from build123d import *

# Parameters (mm, degrees)
F0_W      = 30.48
F0_H      = 15.24
F2_DEPTH  = 3.175
F1_R      = 2.413
F3_DEPTH  = 1.905
F5_R      = 1.27
F6_DEPTH  = 4.699
F4_W      = 27.94
F4_H      = 12.7
F4_R      = 3.175
F7_DEPTH  = 2.159
F8_DEPTH  = 4.699
F9_DEPTH  = 4.699
F4_R_2    = 2.54
F10_DEPTH = 2.159
F11_DEPTH = 2.159
F12_DEPTH = 2.159


with BuildPart() as f2:
    # F0 (on Top) → F2 (new body)
    with BuildSketch(Plane.XY):
        with Locations((-38.230583, 21.220251)):
            Rectangle(F0_W, F0_H)
    extrude(amount=-F2_DEPTH)

    # F1 (on face) → F3 (join)
    with BuildSketch(Plane.XY):
        with Locations((-26.800583, 25.030251)):
            Circle(F1_R)
        with Locations((-26.800583, 17.410251)):
            Circle(F1_R)
        with Locations((-34.420583, 25.030251)):
            Circle(F1_R)
        with Locations((-34.420583, 17.410251)):
            Circle(F1_R)
        with Locations((-42.040583, 25.030251)):
            Circle(F1_R)
        with Locations((-42.040583, 17.410251)):
            Circle(F1_R)
        with Locations((-49.660583, 25.030251)):
            Circle(F1_R)
        with Locations((-49.660583, 17.410251)):
            Circle(F1_R)
    extrude(amount=F3_DEPTH)

    # F5 (on face) → F6 (cut)
    with BuildSketch(Plane(origin=(0, 0, -3.175), x_dir=(1, 0, 0), z_dir=(0, 0, -1))):
        with Locations((-26.800583, -25.030251)):
            Circle(F5_R)
        with Locations((-34.420583, -25.030251)):
            Circle(F5_R)
        with Locations((-42.040583, -25.030251)):
            Circle(F5_R)
        with Locations((-49.660583, -25.030251)):
            Circle(F5_R)
        with Locations((-26.800583, -17.410251)):
            Circle(F5_R)
        with Locations((-34.420583, -17.410251)):
            Circle(F5_R)
        with Locations((-42.040583, -17.410251)):
            Circle(F5_R)
        with Locations((-49.660583, -17.410251)):
            Circle(F5_R)
    extrude(amount=-F6_DEPTH, mode=Mode.SUBTRACT)

    # F4 (on face) → F7 (cut)
    with BuildSketch(Plane(origin=(0, 0, -3.175), x_dir=(1, 0, 0), z_dir=(0, 0, -1))):
        with Locations((-38.230583, -21.220251)):
            Rectangle(F4_W, F4_H)
        with Locations((-45.850583, -21.220251)):
            Circle(F4_R, mode=Mode.SUBTRACT)
        with Locations((-38.230583, -21.220251)):
            Circle(F4_R, mode=Mode.SUBTRACT)
        with Locations((-30.610583, -21.220251)):
            Circle(F4_R, mode=Mode.SUBTRACT)
    extrude(amount=-F7_DEPTH, mode=Mode.SUBTRACT)

    # F5 (on face) → F8 (join)
    with BuildSketch(Plane(origin=(0, 0, -3.175), x_dir=(1, 0, 0), z_dir=(0, 0, -1))):
        with Locations((-49.660583, -25.030251)):
            Circle(F5_R)
    extrude(amount=-F8_DEPTH)

    # F5 (on face) → F9 (cut)
    with BuildSketch(Plane(origin=(0, 0, -3.175), x_dir=(1, 0, 0), z_dir=(0, 0, -1))):
        with Locations((-49.660583, -25.030251)):
            Circle(F5_R)
    extrude(amount=-F9_DEPTH, mode=Mode.SUBTRACT)

    # F4 (on face) → F10 (cut)
    with BuildSketch(Plane(origin=(0, 0, -3.175), x_dir=(1, 0, 0), z_dir=(0, 0, -1))):
        with Locations((-45.850583, -21.220251)):
            Circle(F4_R_2)
    extrude(amount=-F10_DEPTH, mode=Mode.SUBTRACT)

    # F4 (on face) → F11 (cut)
    with BuildSketch(Plane(origin=(0, 0, -3.175), x_dir=(1, 0, 0), z_dir=(0, 0, -1))):
        with Locations((-30.610583, -21.220251)):
            Circle(F4_R_2)
    extrude(amount=-F11_DEPTH, mode=Mode.SUBTRACT)

    # F4 (on face) → F12 (cut)
    with BuildSketch(Plane(origin=(0, 0, -3.175), x_dir=(1, 0, 0), z_dir=(0, 0, -1))):
        with Locations((-38.230583, -21.220251)):
            Circle(F4_R_2)
    extrude(amount=-F12_DEPTH, mode=Mode.SUBTRACT)


solid = f2.part
Build history of the part. All positions in model axes, mm. A direction names the side the tool comes from. Coordinates: 2 decimals unless noted, no trailing zeros. Order: outer loops, then holes, each group sorted by start corner. A loop starts at its lowest first (then second) coordinate and runs counter-clockwise, first axis right, second up. Notation, with made-up numbers: (45, -13) - (95, -13) arc R5 cw to (95, -9) - close; hole circle Ø7 at (70, 43). An arc over 180 degrees is marked (long way). Write each question's results on one line, items separated by ' | '. Start each with the question number.
Item 1: Tool access for faces 4 (the face through (-30, 24, -3.175)), 5 (the face through (-27, 17, 1.524)), 6 (the face through (-44.45, 25.14, 0.94)): list every direction of +Z, -Z, +X, -X, +Y, -Y with a clear straight run to the whole face (end or side of a thin tool).
Item 2: Flat gauge pins, fed straight in: pin 1 (2 mm diameter, centred on x = -31, y = 16.5, fed in from +Z); pin 2 (0.8 mm diameter, centred on x = -49.5, y = 25, fed in from -Z); pin 3 (1.5 mm diameter, centred on x = -45, z = 0.5, fed in from +Y); pin 4 (2.5 mm diameter, centred on x = -37.5, y = 21, fed in from -Z). Where does each tip first touch, or does it go through?
Item 3: Band-saw the part on A-A on z = -2.7. Write the cut outline in (x, y) (3 decimals).
Item 4: Wall check: probe 1 along Y at (x, z) = (-43, -0.8); probe 2 along Y at (x, z) = (-51.5, -1.95); probe 3 along Y at (x, z) = (-35.5, -2.7). Give the ranges that are in metal, low to high. Write a range as [from, to].
Item 5: Band-saw the part on C-C on x = -31. Write the cut outline in (y, z) (3 decimals).
Item 6: Mould opens along Y. For faces 1 (the face through (-44.45, 17.52, 0.94)), 2 (the face through (-32.19, 16.49, 0.94)), 3 (the face through (-42, 17, 1.905)) say: released by +Y, released by -Y, zero draft, split by the parting line, or undercut.
Item 7: Band-saw the part on B-B on z = 1.2. State how many separate pieces and enclosed holes the cut face has, and give its area (3 significant figures).
Numbers:
1) face 4: -Z, +X, -X, +Y, -Y | face 5: -Z | face 6: +Z
2) pin 1: z = 0 | pin 2: z = 1.52 | pin 3: y = 28.84 | pin 4: z = -1.02
3) outline: (-53.471, 13.6) - (-22.991, 13.6) - (-22.991, 28.84) - (-53.471, 28.84) - close; circle Ø6.35 at (-45.851, 21.22); circle Ø6.35 at (-38.231, 21.22); circle Ø6.35 at (-30.611, 21.22); hole (-52.201, 14.87) - (-24.261, 14.87) - (-24.261, 27.57) - (-52.201, 27.57) - close; hole circle Ø5.08 at (-45.851, 21.22); hole circle Ø5.08 at (-38.231, 21.22); hole circle Ø5.08 at (-30.611, 21.22)
4) probe 1: [13.6, 16.58], [18.24, 24.2], [25.86, 28.84] | probe 2: [13.6, 14.87], [27.57, 28.84] | probe 3: [13.6, 14.87], [19.6, 22.84], [27.57, 28.84]
5) outline: (13.6, -3.175) - (14.87, -3.175) - (14.87, -1.016) - (18.069, -1.016) - (18.069, -3.175) - (18.71, -3.175) - (18.71, -1.016) - (23.73, -1.016) - (23.73, -3.175) - (24.371, -3.175) - (24.371, -1.016) - (27.57, -1.016) - (27.57, -3.175) - (28.84, -3.175) - (28.84, 0) - (13.6, 0) - close
6) face 1: undercut | face 2: undercut | face 3: zero draft
7) separate pieces: 8 | enclosed holes: 8 | area: 106 mm^2
